Geometry check sheet. Reference: the model listing, model coordinates, mm. A direction names the side the tool comes from. Give positions to 0.01 mm unless a question says otherwise; leave off trailing zeros. Write each loop counter-clockwise with the first axis right and the second up, starting at its lowest first coordinate (ties: lowest second). Pieces come first, ordered by that corner, then holes. Notation, with made-up numbers: (-15.75, 49.5) - (26.25, 49.5) arc R11 cw to (26.25, 64.5) - close; hole circle Ø5 at (22, 65.5). An arc over 180 degrees is marked (long way). One line per question, with ' | ' between items. Start each with the question number.
Q1. Thickness scan on L1, parallel to X at y = 3.1, z = -1.2; L2, parallel to X at y = 2.5, z = -17.25; L3, parallel to X at y = 1.65, z = -18.8. Record the ranges inside material, lowest first. Write a range as [from, to].
Q2. Section check D-D on x = 8. Record the boundary of the cut face in (y, z), and give its area (3 significant figures).
Q3. Section check B-B on z = -18.8. Record the boundary of the cut face in (x, y).
Q4. Section check A-A on x = 12.3. Record the boundary of the cut face in (y, z).
Q5. Set-up check for faces 4 (the face through (16.25, 2, -9)), 5 (the face through (6.8, 2, -12.5)), 6 (the face through (6.5, 1.5, -2)): record each of +Z, -Z, +X, -X, +Y, -Y from which the full face is reachable in a straight line by a thin tool's end or side.
Q6. Section check C-C on y = 2.95. Count the separate pieces of the cut face and the enclosed holes in it, and give its area (3 significant figures).
Q7. Gauge pin test, flat ends, axial feed: P1, Ø0.8, axis at x = 8, y = 1.5, coming from the +Z side; P2, Ø5.5, axis at x = 7, z = 3.5, coming from the +Y side; P3, Ø2, axis at x = 8, z = -1, coming from the +Y side. Record the tip position at first contact, or that the pin passes through.
Q8. Release check for a two-part mould opening along Z. For faces 1 (the face through (3, 4, -12)), 2 (the face through (9.25, 2, -15)), 3 (the face through (6.7, 1.5, 0)) record: +Z half, -Z half, draft (parallel to the pull), parting line (faces both ways), or undercut.
```python
from build123d import *

# Parameters (mm, degrees)
SKETCH1_W           = 13.5
SKETCH1_H           = 20
BOSS_EXTRUDE1_DEPTH = 1
BOSS_EXTRUDE2_DEPTH = 3
BOSS_EXTRUDE3_DEPTH = 1
CUT_EXTRUDE1_START  = -1
SKETCH4_R           = 0.7
CUT_EXTRUDE1_DEPTH  = 11.5
SKETCH5_W           = 9.5
SKETCH5_H           = 2
BOSS_EXTRUDE4_DEPTH = 1
SKETCH6_W           = 19
SKETCH6_H           = 28
SKETCH6_W_2         = 13.5
SKETCH6_H_2         = 20
BOSS_EXTRUDE5_DEPTH = 1
BOSS_EXTRUDE6_DEPTH = 3


with BuildPart() as part:
    # Sketch1 → Boss-Extrude1 (new body)
    with BuildSketch(Plane(origin=(0, 0, 0), x_dir=(1, 0, 0), z_dir=(0, 1, 0))):
        with Locations((6.75, 10)):
            Rectangle(SKETCH1_W, SKETCH1_H)
    extrude(amount=BOSS_EXTRUDE1_DEPTH)

    # Sketch2 → Boss-Extrude2 (add)
    with BuildSketch(Plane(origin=(0, 1, 0), x_dir=(1, 0, 0), z_dir=(0, 1, 0))):
        with BuildLine():
            Line((2, 10), (2, 2))
            Line((2, 2), (2, 0))
            Line((2, 0), (0, 0))
            Line((0, 0), (0, 20))
            Line((0, 20), (13.5, 20))
            Line((13.5, 20), (13.5, 0))
            Line((13.5, 0), (11.5, 0))
            add(Edge.make_bspline(
                [(11.5, 2.535585729), (10.536627545, 1.300187459), (11.5, 0)],
                knots=[0, 0, 0, 1, 1, 1], degree=2))
            Line((11.5, 2.535585729), (11.5, 10))
            Line((11.5, 10), (9.25, 13))
            Line((9.25, 13), (9.25, 18))
            Line((9.25, 18), (4.25, 18))
            Line((4.25, 18), (4.25, 13))
            Line((4.25, 13), (2, 10))
        make_face()
    extrude(amount=BOSS_EXTRUDE2_DEPTH)

    # Sketch3 → Boss-Extrude3 (add)
    with BuildSketch(Plane(origin=(0, 1, 0), x_dir=(1, 0, 0), z_dir=(0, 1, 0))):
        Polygon((4.25, 13), (9.25, 13), (10, 12), (3.5, 12), align=None)
    extrude(amount=BOSS_EXTRUDE3_DEPTH)

    # Sketch4 → Cut-Extrude1 (cut)
    with BuildSketch(Plane.XZ.offset(CUT_EXTRUDE1_START)):
        with Locations(Location((1.2, -18.8, 0), (0, 0, 270))):
            Circle(SKETCH4_R)
        with Locations(Location((12.3, -1.2, 0), (0, 0, 270))):
            Circle(SKETCH4_R)
    extrude(amount=-CUT_EXTRUDE1_DEPTH, mode=Mode.SUBTRACT)

    # Sketch5 → Boss-Extrude4 (add)
    with BuildSketch(Plane(origin=(0, 1, 0), x_dir=(1, 0, 0), z_dir=(0, 1, 0))):
        with Locations((6.75, 1)):
            Rectangle(SKETCH5_W, SKETCH5_H)
    extrude(amount=BOSS_EXTRUDE4_DEPTH)

    # Sketch6 → Boss-Extrude5 (add)
    with BuildSketch(Plane(origin=(0, 1, 0), x_dir=(1, 0, 0), z_dir=(0, 1, 0))):
        with Locations((6.75, 9)):
            Rectangle(SKETCH6_W, SKETCH6_H)
        with Locations((6.75, 10)):
            Rectangle(SKETCH6_W_2, SKETCH6_H_2, mode=Mode.SUBTRACT)
    extrude(amount=-BOSS_EXTRUDE5_DEPTH)

    # Sketch7 → Boss-Extrude6 (add)
    with BuildSketch(Plane(origin=(0, 4, 0), x_dir=(1, 0, 0), z_dir=(0, 1, 0))):
        Polygon((2, 0), (2, -5), (-2.75, -5), (-2.75, 23), (16.25, 23), (16.25, -5), (11.5, -5), (11.5, 0), (13.5, 0), (13.5, 20), (0, 20), (0, 0), align=None)
    extrude(amount=-BOSS_EXTRUDE6_DEPTH)


solid = part.part
```
Working result:
1) L1: x = [-2.75, 2], [11.02, 11.6], [13, 16.25] | L2: x = [-2.75, 4.25], [9.25, 16.25] | L3: x = [-2.75, 0.5], [1.9, 16.25]
2) outline: (0, -23) - (4, -23) - (4, -18) - (1, -18) - (1, -13) - (2, -13) - (2, -12) - (1, -12) - (1, -2) - (2, -2) - (2, 0) - (1, 0) - (1, 5) - (0, 5) - close | area: 46.0 mm2
3) outline: (-2.75, 0) - (16.25, 0) - (16.25, 4) - (1.9, 4) - (1.9, 1) - (0.5, 1) - (0.5, 4) - (-2.75, 4) - close
4) outline: (0, -23) - (4, -23) - (4, -1.9) - (1, -1.9) - (1, -0.5) - (4, -0.5) - (4, 5) - (0, 5) - close
5) face 4: +Z, -Z, +X, +Y, -Y | face 5: +Z, +Y | face 6: +Y
6) separate pieces: 1 | enclosed holes: 2 | area: 340 mm2
7) P1: stops at z = 0 | P2: stops at y = 1 | P3: stops at y = 2
8) face 1: draft | face 2: undercut | face 3: +Z half
